Source: three-view drawing plus pictorial views. Frame: mm from the lowest corner of the part. A direction names the side the tool comes from. Round coordinates to 2 decimals unless told otherwise and drop trailing zeros. Loops run counter-clockwise (first coordinate to the right, second up) from the corner with the lowest first, then second, coordinate; pieces in that order, holes last. Notation, with made-up numbers: (22, -36) -> (81, -36) arc R30 cw to (81, -6) -> close; hole circle Ø6 at (-7.5, -24). An arc over 180 degrees is marked (long way). Answer as a JSON object with one key per item and string values. Group by question number.
Item 1: Section query A-A on y = 26. Return loops of the section in (x, z) (1 decimal), and give its area (3 significant figures).
Item 2: Material intervals for line 1 (Z direction, x = 24.5, y = 28) (1 decimal); line 2 (Y direction, x = 5.5, z = 22), sorted ascending. Write a range as [from, to].
Item 3: Section query D-D on z = 103.5. Return loops of the section in (x, y).
Item 4: Set-up query: the marked faces 4 and 5. Return all of +Z, -Z, +X, -X, +Y, -Y with unobstructed straight access to the full face (end or side cutting, diameter ignored); none if empty.
Item 5: Section query B-B on x = 5.5. Return loops of the section in (y, z) (1 decimal).
Item 6: Draft query along Z for the marked faces 1, 2 and 3. Return one class per face: released by +Z, released by -Z, zero draft, split by the parting line, or undercut.
Item 7: Pin query (flat end, axial travel): pin 1 (11.5 mm diameter, centred on x = 17, z = 72.5, fed in from +Y). Return the tip coordinate at first contact, or that it passes through.
Item 8: Section query C-C on x = 16.5. Return loops of the section in (y, z) (1 decimal).
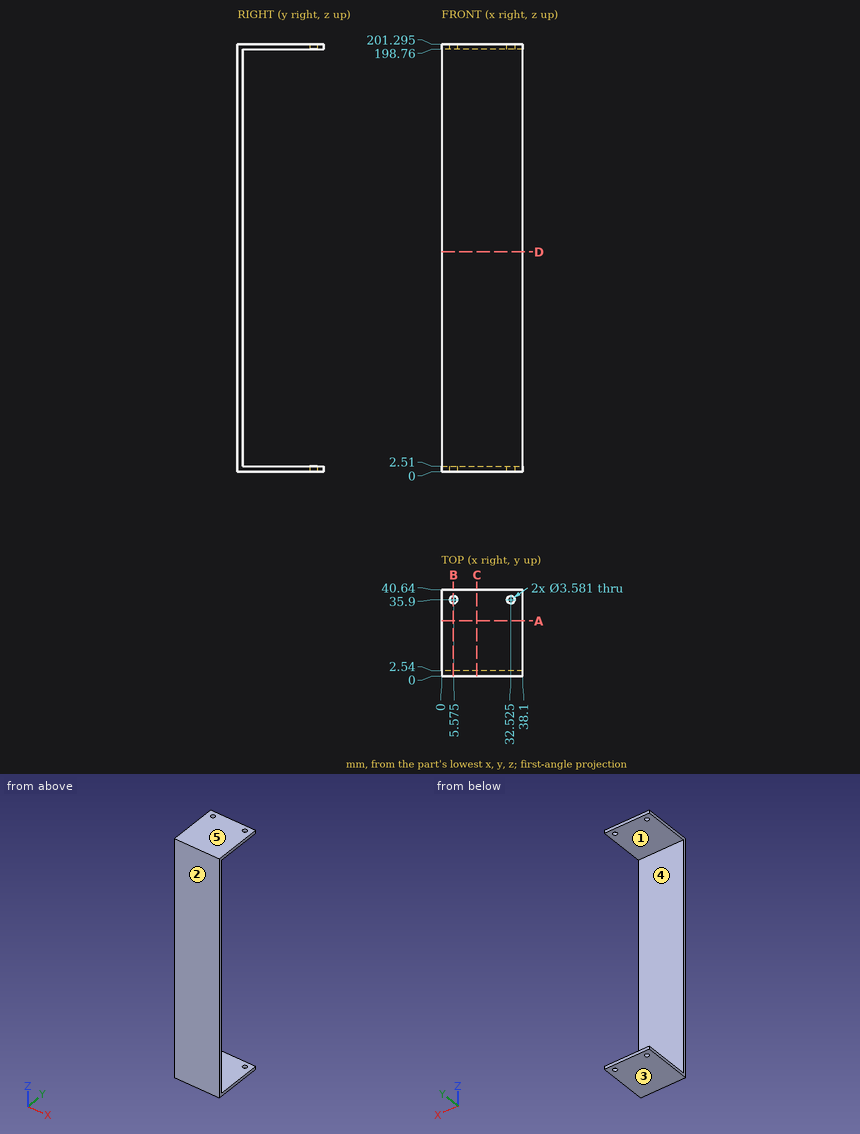
Solved:
{
 "1": {"outline": "(0, 0) -> (38.1, 0) -> (38.1, 2.5) -> (0, 2.5) -> close; (0, 198.8) -> (38.1, 198.8) -> (38.1, 201.3) -> (0, 201.3) -> close", "area": "192 mm²"},
 "2": {"line 1": "[0, 2.5], [198.8, 201.3]", "line 2": "[0, 2.54]"},
 "3": {"outline": "(0, 0) -> (38.1, 0) -> (38.1, 2.54) -> (0, 2.54) -> close"},
 "4": {"face 4": "+X, -X, +Y", "face 5": "+Z, +X, -X, +Y, -Y"},
 "5": {"outline": "(0, 0) -> (34.1, 0) -> (34.1, 2.5) -> (2.5, 2.5) -> (2.5, 198.8) -> (34.1, 198.8) -> (34.1, 201.3) -> (0, 201.3) -> close; (37.7, 0) -> (40.6, 0) -> (40.6, 2.5) -> (37.7, 2.5) -> close; (37.7, 198.8) -> (40.6, 198.8) -> (40.6, 201.3) -> (37.7, 201.3) -> close"},
 "6": {"face 1": "undercut", "face 2": "zero draft", "face 3": "released by -Z"},
 "7": {"pin 1": "y = 2.54"},
 "8": {"outline": "(0, 0) -> (40.6, 0) -> (40.6, 2.5) -> (2.5, 2.5) -> (2.5, 198.8) -> (40.6, 198.8) -> (40.6, 201.3) -> (0, 201.3) -> close"}
}
